Autodesk Inventor part; units mm, degrees
ref_plane "ANBAU_XY" through (0, 0, 0) normal (0, 0, -1) x (1, 0, 0)
ref_plane "ANBAU_YZ" through (0, 0, 0) normal (1, 0, 0) x (0, -1, 0)
ref_plane "ANBAU_ZX" through (0, 0, 0) normal (0, -1, 0) x (0, 0, -1)
sketch "Sketch_1" plane through (0, 0, 0) normal (0, 0, 1) x (1, 0, 0)
  line L0 (-2.5, 4.0386) -> (-2.5, 0)
  line L1 (-2.5, 0) -> (2.5, 0)
  line L2 (2.5, 0) -> (2.5, 4.0386)
  arc A0 (2.5, 4.0386) -> (2.3613, 4.229) centre (2.3, 4.0386) ccw
  arc A1 (2.3613, 4.229) -> (-2.3613, 4.229) centre (0, -3.1) ccw
  arc A2 (-2.3613, 4.229) -> (-2.5, 4.0386) centre (-2.3, 4.0386) ccw
extrude "Extrusion1" add sketch "Sketch_1" along normal blind 26.3
sketch "Sketch_2" plane through (-1.6, 0, 0) normal (1, 0, 0) x (0, 0, -1)
  line L0 (-15.3, 3.85) -> (-15.3, 2)
  line L1 (-15.3, 2) -> (-10.025, 2)
  line L2 (-10.025, 2) -> (-10.025, 3.15)
  line L3 (-10.025, 3.15) -> (-10.725, 3.15)
  line L4 (-10.725, 3.15) -> (-10.725, 3.85)
  line L5 (-10.725, 3.85) -> (-15.3, 3.85)
extrude "Extrusion2" cut sketch "Sketch_2" along normal blind 4.1
sketch "Sketch_3" plane through (-2.5, 0, 0) normal (1, 0, 0) x (0, 0, -1)
  line L0 (-16.875, 3.85) -> (-16.875, 2)
  line L1 (-16.875, 2) -> (-11.6, 2)
  line L2 (-11.6, 2) -> (-11.6, 3.85)
  line L3 (-11.6, 3.85) -> (-16.875, 3.85)
extrude "Extrusion3" cut sketch "Sketch_3" along normal blind 4.1
sketch "Sketch_4" plane through (0, 4.6, 0) normal (0, 1, 0) x (1, 0, 0)
  line L0 (-3, -15.3) -> (-1.3666, -15.3)
  arc A0 (-1.3666, -15.3) -> (1.3666, -15.3) centre (0, -13.45) ccw
  line L1 (1.3666, -15.3) -> (3, -15.3)
  line L2 (3, -15.3) -> (3, -11.6)
  line L3 (3, -11.6) -> (1.3666, -11.6)
  arc A1 (1.3666, -11.6) -> (-1.3666, -11.6) centre (0, -13.45) ccw
  line L4 (-1.3666, -11.6) -> (-3, -11.6)
  line L5 (-3, -11.6) -> (-3, -15.3)
extrude "Extrusion4" cut sketch "Sketch_4" against normal blind 2.5
sketch "Sketch_5" plane through (0, 2, 0) normal (0, 1, 0) x (1, 0, 0)
  arc A0 (-2.6719, -11.644) -> (-2.6719, -15.256) centre (0, -13.45) ccw
  arc A1 (-2.6719, -15.256) -> (-2.589, -15.3) centre (-2.589, -15.2) ccw
  line L0 (-2.589, -15.3) -> (-1.9442, -15.3)
  arc A2 (-1.6255, -15.4148) -> (-1.9442, -15.3) centre (-1.9442, -15.8) ccw
  arc A3 (-1.6255, -15.4148) -> (1.6255, -15.4148) centre (0, -13.45) ccw
  arc A4 (1.9442, -15.3) -> (1.6255, -15.4148) centre (1.9442, -15.8) ccw
  line L1 (1.9442, -15.3) -> (2.589, -15.3)
  arc A5 (2.589, -15.3) -> (2.6719, -15.256) centre (2.589, -15.2) ccw
  arc A6 (2.6719, -15.256) -> (2.6719, -11.644) centre (0, -13.45) ccw
  arc A7 (2.6719, -11.644) -> (2.589, -11.6) centre (2.589, -11.7) ccw
  line L2 (2.589, -11.6) -> (1.9442, -11.6)
  arc A8 (1.6255, -11.4852) -> (1.9442, -11.6) centre (1.9442, -11.1) ccw
  arc A9 (1.6255, -11.4852) -> (-1.6255, -11.4852) centre (0, -13.45) ccw
  arc A10 (-1.9442, -11.6) -> (-1.6255, -11.4852) centre (-1.9442, -11.1) ccw
  line L3 (-1.9442, -11.6) -> (-2.589, -11.6)
  arc A11 (-2.589, -11.6) -> (-2.6719, -11.644) centre (-2.589, -11.7) ccw
extrude "Extrusion5" add sketch "Sketch_5" along normal blind 1
sketch "Sketch_6" plane through (0, 0, 13.45) normal (0, 0, 1) x (1, 0, 0)
  line L0 (0, 2) -> (0, 4.6)
  line L1 (0, 4.6) -> (2.25, 4.6)
  line L2 (2.25, 4.6) -> (2.25, 3.9)
  line L3 (2.25, 3.9) -> (1.6935, 3.9)
  line L4 (1.6935, 3.9) -> (1.6935, 3.6)
  line L5 (1.6935, 3.6) -> (2, 3.2935)
  line L6 (2, 3.2935) -> (2, 2.3065)
  line L7 (2, 2.3065) -> (1.6935, 2)
  line L8 (1.6935, 2) -> (0, 2)
  line L9 (0, 2) -> (0, 4.6)
revolve "Revolution1" add sketch "Sketch_6" angle 360 about axis through (0, 2, 13.45) along (0, -1, 0)
thread "Thread1"
sketch "Sketch_7" plane through (0, 4.6, 13.45) normal (0, 1, 0) x (1, 0, 0)
  line L0 (-0.75, -0.433) -> (0, -0.866)
  line L1 (0, -0.866) -> (0.75, -0.433)
  line L2 (0.75, -0.433) -> (0.75, 0.433)
  line L3 (0.75, 0.433) -> (0, 0.866)
  line L4 (0, 0.866) -> (-0.75, 0.433)
  line L5 (-0.75, 0.433) -> (-0.75, -0.433)
extrude "Extrusion6" cut sketch "Sketch_7" against normal blind 1.4
sketch "Sketch_9" plane through (0, 0, 23.21) normal (0, 0, 1) x (1, 0, 0)
  line L0 (-2.5, 2.8) -> (2.5, 2.8)
  line L1 (2.5, 2.8) -> (2.5, 4.2485)
  arc A0 (2.5, 4.2485) -> (2.3597, 4.4393) centre (2.3, 4.2485) ccw
  arc A1 (2.3597, 4.4393) -> (-2.3597, 4.4393) centre (0, -3.1) ccw
  arc A2 (-2.3597, 4.4393) -> (-2.5, 4.2485) centre (-2.3, 4.2485) ccw
  line L2 (-2.5, 4.2485) -> (-2.5, 2.8)
extrude "Extrusion7" add sketch "Sketch_9" along normal mid plane 0.4
sketch "Sketch_10" plane through (0, 0, 23.21) normal (0, 0, 1) x (1, 0, 0)
  line L0 (-0.2, 2.78) -> (0.2, 2.78)
  line L1 (0.2, 2.78) -> (0.2, 4.78)
  line L2 (0.2, 4.78) -> (-0.2, 4.78)
  line L3 (-0.2, 4.78) -> (-0.2, 2.78)
extrude "Extrusion8" add sketch "Sketch_10" along normal mid plane 2
sketch "Sketch_11" plane through (0, 0, 0) normal (1, 0, 0) x (0, 1, 0)
  line L0 (2.05, -90) -> (2.05, 0)
  line L1 (2.05, 0) -> (4.05, 0)
  line L2 (4.05, 0) -> (4.05, -3)
  line L3 (4.05, -3) -> (3.5, -3)
  line L4 (3.5, -3) -> (3.5, -90)
  line L5 (3.5, -90) -> (2.05, -90)
  line L6 (2.05, -90) -> (2.05, 0)
revolve "Revolution2" add sketch "Sketch_11" angle 360 about axis through (0, 2.05, -90) along (0, 0, -1)
sketch "Sketch_12" plane through (0, 2.05, -90) normal (0, 0, -1) x (0, 1, 0)
  line L0 (-2, -2) -> (2, -2)
  line L1 (2, -2) -> (2, 2)
  line L2 (2, 2) -> (-2, 2)
  line L3 (-2, 2) -> (-2, -2)
  circle A0 centre (0.4, 0) radius 0.3
  circle A1 centre (-0.2, 0.3464) radius 0.3
  circle A2 centre (-0.2, -0.3464) radius 0.3
extrude "Extrusion9" cut sketch "Sketch_12" against normal blind 10
sketch "Sketch_17" plane through (0, 0, -1.5) normal (0, 0, 1) x (1, 0, 0)
  arc A0 (-3.0691, 2.4416) -> (-2.9069, 2.2099) centre (-2.8722, 2.4069) ccw
  line L0 (-2.9069, 2.2099) -> (0, 1.6973)
  line L1 (0, 1.6973) -> (2.9069, 2.2099)
  arc A1 (2.9069, 2.2099) -> (3.0691, 2.4416) centre (2.8722, 2.4069) ccw
  line L2 (3.0691, 2.4416) -> (3.0531, 2.5326)
  arc A2 (3.0531, 2.5326) -> (2.8214, 2.6948) centre (2.8561, 2.4979) ccw
  line L3 (2.8214, 2.6948) -> (0, 2.1973)
  line L4 (0, 2.1973) -> (-2.8214, 2.6948)
  arc A3 (-2.8214, 2.6948) -> (-3.0531, 2.5326) centre (-2.8561, 2.4979) ccw
  line L5 (-3.0531, 2.5326) -> (-3.0691, 2.4416)
extrude "Extrusion10" add sketch "Sketch_17" along normal mid plane 1.8
ref_plane "ANBAU_XY" through (0, 0, 0) normal (0, 0, -1) x (1, 0, 0)
ref_plane "ANBAU_YZ" through (0, 0, 0) normal (1, 0, 0) x (0, -1, 0)
ref_plane "ANBAU_ZX" through (0, 0, 0) normal (0, -1, 0) x (0, 0, -1)
ref_plane "ASCF1_XY" through (0, 2.05, -10) normal (0, 0, -1) x (1, 0, 0)
ref_plane "ASCF1_YZ" through (0, 2.05, -10) normal (1, 0, 0) x (0, -1, 0)
ref_plane "ASCF1_ZX" through (0, 2.05, -10) normal (0, -1, 0) x (0, 0, -1)
ref_plane "ASCF2_XY" through (0, 2.05, -75) normal (0, 0, 1) x (1, 0, 0)
ref_plane "ASCF2_YZ" through (0, 2.05, -75) normal (1, 0, 0) x (0, 1, 0)
ref_plane "ASCF2_ZX" through (0, 2.05, -75) normal (0, 1, 0) x (0, 0, 1)
ref_plane "FDT_NUT_XY" through (0, 0, 26.3) normal (0, -1, 0) x (1, 0, 0)
ref_plane "FDT_NUT_YZ" through (0, 0, 26.3) normal (1, 0, 0) x (0, 0, 1)
ref_plane "FDT_NUT_ZX" through (0, 0, 26.3) normal (0, 0, 1) x (0, -1, 0)
properties part number "574333 SMT-8M-A-1---OE---(part)"
Model file for the job. Use its own axes, mm. A direction names the side the tool comes from. Coordinates: 2 decimals unless noted, no trailing zeros. Write each loop counter-clockwise with the first axis right and the second up, starting at its lowest first coordinate (ties: lowest second). Pieces come first, ordered by that corner, then holes. Notation, with made-up numbers: (75.5, 7.5) - (116.5, 7.5) arc R30 ccw to (116.5, 32.5) - close; hole circle Ø1 at (41, -11.75). An arc over 180 degrees is marked (long way). Use a Markdown table: item, result. Add a question column.
Item 1: 3-axis set-ups, long thin cutter, end or side, ignore diameter. For faces 1 (the face through (0, 4.6, 5.7)), 2 (the face through (0, 3, 16.875)), 3 (the face through (-1, 2, -80)), 4 (the face through (0, 4.6, 12)): which of +Z, -Z, +X, -X, +Y, -Y reach the whole face in a straight line?
Item 2: Drill centre lines: line 1 along Z through (x, y) = (2.75, 2.25); line 2 along Z through (x, y) = (1.5, 4.5); line 3 along X through (y, z) = (2.1, -64.5). Where is each one in solid material? Low to high.
Item 3: Drop flat-ended pins along their axis: pin 1 (1 mm diameter, centred on y = 4, z = 13.5, fed in from +X); pin 2 (3.5 mm diameter, centred on x = -1, z = 12.5, fed in from -Y); pin 3 (0.9 mm diameter, centred on x = -1.5, y = 2.5, fed in from -Z); pin 4 (1.5 mm diameter, centred on y = 3.5, z = -47, fed in from -X). Give the stop position or say it passes through.
Item 4: Band-saw the part on A-A, the plane z = -55.5. Write the cut outline in (x, y).
Item 5: Two-plate mould, pull along Z, no slides. Class faces 5 (the face through (0, 2, 26.3)), 6 (the face through (-2.2, 3, 13.4)), 7 (the face through (0.44, 3.43, -42.04)): pulls with the +Z half, pulls with the -Z half, needs draft (parallel to the pull), parting line crosses it, or undercut.
A:
| question | item | result |
|---|---|---|
| 1 | face 1 | -Z, +Y |
| 1 | face 2 | -X |
| 1 | face 3 | -Z |
| 1 | face 4 | -Z, +X, -X, +Y |
| 2 | line 1 | z = -2.4 to -0.6, 11.77 to 15.13 |
| 2 | line 2 | z = 11.77 to 15.13, 23.01 to 23.41 |
| 2 | line 3 | x = -1.45 to 1.45 |
| 3 | pin 1 | stops at x = 2.25 |
| 3 | pin 2 | stops at y = 0 |
| 3 | pin 3 | stops at z = -80 |
| 3 | pin 4 | stops at x = -1.27 |
| 4 | outline | circle Ø2.9 at (0, 2.05) |
| 5 | face 5 | pulls with the +Z half |
| 5 | face 6 | undercut |
| 5 | face 7 | needs draft |
